The model under review builds one solid part; all positions refer to its coordinate system, in mm. Coordinates: 2 decimals unless noted, no trailing zeros. Order: outer loops, then holes, each group sorted by start corner. A loop starts at its lowest first (then second) coordinate and runs counter-clockwise, first axis right, second up.
```python
from build123d import *

# Parameters (mm, degrees)
SKETCH_1_R          = 11
EXTRUDE_1_DEPTH     = 20
SKETCH_2_R          = 11
EXTRUDE_2_DEPTH     = 480
SKETCH_4_R          = 9
CUT_EXTRUDE_1_DEPTH = 501


with BuildPart() as part:
    # 草图1 → 凸台-拉伸1 (new body)
    with BuildSketch(Plane(origin=(0, 0, 0), x_dir=(1, 0, 0), z_dir=(0, 1, 0))):
        Circle(SKETCH_1_R)
    extrude(amount=EXTRUDE_1_DEPTH)

    # 草图2 → 凸台-拉伸2 (add)
    with BuildSketch(Plane(origin=(0, 20, 0), x_dir=(1, 0, 0), z_dir=(0, 1, 0))):
        Circle(SKETCH_2_R)
    extrude(amount=EXTRUDE_2_DEPTH)

    # 草图4 → 切除-拉伸1 (cut, through all)
    with BuildSketch(Plane.XZ):
        Circle(SKETCH_4_R)
    extrude(amount=-CUT_EXTRUDE_1_DEPTH, mode=Mode.SUBTRACT)


solid = part.part
```
(1) We need section A-A, the plane z = 0. Write out the cut boundary in (x, y).
A:
outline: (-11, 0) - (-9, 0) - (-9, 500) - (-11, 500) - close; (9, 0) - (11, 0) - (11, 500) - (9, 500) - close
(2) Draft analysis for pull direction Z (two halves, no side actions). For faces 1 (the face through (2, 500, 9)), 2 (the face through (-1.172, 246.5, 8.923)), 3 (the face through (-2.38, 246.5, 10.74)), state which applies: released by +Z, released by -Z, zero draft, split by the parting line, or undercut.
A:
face 1: zero draft
face 2: undercut
face 3: split by the parting line
(3) Wall thickness on probe 1 along Z at (x, y) = (0, 332); probe 2 along X at (y, z) = (173.5, -7); probe 3 along Z at (x, y) = (6.75, 430): over which ranges is each line inside the solid? List them lowest first.
A:
probe 1: z = -11 to -9, 9 to 11
probe 2: x = -8.49 to -5.66, 5.66 to 8.49
probe 3: z = -8.69 to -5.95, 5.95 to 8.69
(4) We need section B-B, the plane x = 0. Write out the cut boundary in (y, z).
A:
outline: (0, -11) - (500, -11) - (500, -9) - (0, -9) - close; (0, 9) - (500, 9) - (500, 11) - (0, 11) - close
(5) For pin 1 Ø3 at (y, z) = (263.5, -8) entering from -X; pin 2 Ø3 at (y, z) = (407, -3.5) entering from -X; pin 3 Ø8 at (y, z) = (248.5, -3) entering from +X; pin 4 Ø6 at (x, y) = (-7, 254.5) entering from -Z, all flat-tipped, find the tip position at first contact; note any pin that passes through.
A:
pin 1: stops at x = -8.87
pin 2: stops at x = -10.82
pin 3: stops at x = 11
pin 4: stops at z = -10.25
(6) We need section C-C, the plane y = 391. Write out the cut boundary in (x, z), and give its area (3 significant figures).
A:
outline: circle Ø22 at (0, 0); hole circle Ø18 at (0, 0)
area: 126 mm2
